Model file for the job. Use its own axes, mm. Face numbers are marked on the shaded views. A direction names the side the tool comes from. Coordinates: 2 decimals unless noted, no trailing zeros. Write each loop counter-clockwise with the first axis right and the second up, starting at its lowest first coordinate (ties: lowest second). Pieces come first, ordered by that corner, then holes. Notation, with made-up numbers: M -12.75,43.5 L 43.25,43.5 A19 cw 43.25,49.5 Z; hole C 25.25,39 d1. An arc over 180 degrees is marked long. Answer in a Markdown table with one row per item. Add a question column.
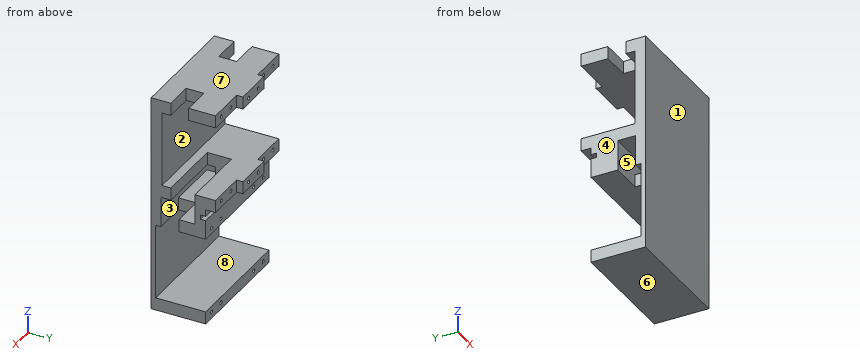
```python
from build123d import *

# Parameters (mm, degrees)
SKETCH1_W            = 66
SKETCH1_H            = 56
BOSS_EXTRUDE1_DEPTH  = 6
SKETCH2_W            = 66
SKETCH2_H            = 7
BOSS_EXTRUDE2_DEPTH  = 30
SKETCH4_W            = 22
SKETCH4_H            = 7
BOSS_EXTRUDE3_DEPTH  = 3.5
SKETCH6_R            = 1
CUT_EXTRUDE1_DEPTH   = 10
SKETCH15_W           = 66
SKETCH15_H           = 66
BOSS_EXTRUDE4_DEPTH  = 2.5
SKETCH16_W           = 66
SKETCH16_H           = 7
BOSS_EXTRUDE6_DEPTH  = 28
SKETCH17_R           = 1
CUT_EXTRUDE2_DEPTH   = 10
CUT_EXTRUDE3_REACH   = 9
SKETCH14_W           = 16
SKETCH14_H           = 10
CUT_EXTRUDE4_REACH   = 75
SKETCH19_W           = 18
SKETCH19_H           = 10
SKETCH24_W           = 66
SKETCH24_H           = 15
BOSS_EXTRUDE9_DEPTH  = 10
SKETCH27_W           = 38
SKETCH27_H           = 13.5
CUT_EXTRUDE9_DEPTH   = 17
SKETCH26_W           = 66
SKETCH26_H           = 3
BOSS_EXTRUDE10_DEPTH = 10
SKETCH28_W           = 66
SKETCH28_H           = 2.5
CUT_EXTRUDE10_DEPTH  = 3


with BuildPart() as part:
    # Sketch1 → Boss-Extrude1 (new body)
    with BuildSketch(Plane(origin=(0, 0, 0), x_dir=(1, 0, 0), z_dir=(0, 1, 0))):
        with Locations((33, 28)):
            Rectangle(SKETCH1_W, SKETCH1_H)
    boss_extrude1 = extrude(amount=BOSS_EXTRUDE1_DEPTH)

    # Sketch2 → Boss-Extrude2 (add)
    with BuildSketch(Plane(origin=(0, 6, 0), x_dir=(1, 0, 0), z_dir=(0, 1, 0))):
        with Locations((33, 52.5)):
            Rectangle(SKETCH2_W, SKETCH2_H)
    boss_extrude2 = extrude(amount=BOSS_EXTRUDE2_DEPTH)

    # Sketch4 → Boss-Extrude3 (add)
    with BuildSketch(Plane(origin=(0, 36, 0), x_dir=(1, 0, 0), z_dir=(0, 1, 0))):
        with Locations((33, 52.5)):
            Rectangle(SKETCH4_W, SKETCH4_H)
    boss_extrude3 = extrude(amount=BOSS_EXTRUDE3_DEPTH)

    # Sketch6 → Cut-Extrude1 (cut, symmetric)
    with BuildSketch(Plane(origin=(0, 36, 0), x_dir=(1, 0, 0), z_dir=(0, 1, 0))):
        with Locations((6, 52.25)):
            Circle(SKETCH6_R)
        with Locations((16, 52.25)):
            Circle(SKETCH6_R)
        with Locations((38, 52.25)):
            Circle(SKETCH6_R)
        with Locations((28, 52.25)):
            Circle(SKETCH6_R)
        with Locations((60, 52.25)):
            Circle(SKETCH6_R)
        with Locations((50, 52.25)):
            Circle(SKETCH6_R)
    cut_extrude1 = extrude(amount=CUT_EXTRUDE1_DEPTH, both=True, mode=Mode.SUBTRACT)

    # Mirror1: Boss-Extrude1, Boss-Extrude2, Boss-Extrude3, Cut-Extrude1 across plane
    add(boss_extrude1.mirror(Plane.XY.offset(-28)))
    add(boss_extrude2.mirror(Plane.XY.offset(-28)))
    add(boss_extrude3.mirror(Plane.XY.offset(-28)))
    add(cut_extrude1.mirror(Plane.XY.offset(-28)), mode=Mode.SUBTRACT)

    # Sketch15 → Boss-Extrude4 (add)
    with BuildSketch(Plane(origin=(0, 0, 0), x_dir=(1, 0, 0), z_dir=(0, 1, 0))):
        with Locations((33, 89)):
            Rectangle(SKETCH15_W, SKETCH15_H)
    extrude(amount=BOSS_EXTRUDE4_DEPTH)

    # Sketch16 → Boss-Extrude6 (add)
    with BuildSketch(Plane(origin=(0, 2.5, 0), x_dir=(1, 0, 0), z_dir=(0, 1, 0))):
        with Locations((33, 69.5)):
            Rectangle(SKETCH16_W, SKETCH16_H)
    boss_extrude6 = extrude(amount=BOSS_EXTRUDE6_DEPTH)

    # Sketch17 → Cut-Extrude2 (cut)
    with BuildSketch(Plane(origin=(0, 30.5, 0), x_dir=(1, 0, 0), z_dir=(0, 1, 0))):
        with Locations((6, 69.75)):
            Circle(SKETCH17_R)
        with Locations((16, 69.75)):
            Circle(SKETCH17_R)
        with Locations((50, 69.75)):
            Circle(SKETCH17_R)
        with Locations((60, 69.75)):
            Circle(SKETCH17_R)
    cut_extrude2 = extrude(amount=-CUT_EXTRUDE2_DEPTH, mode=Mode.SUBTRACT)

    # Mirror2: Boss-Extrude6, Cut-Extrude2 across plane
    add(boss_extrude6.mirror(Plane(origin=(0, 0, -94), x_dir=(1, 0, 0), z_dir=(0, 0, -1))))
    add(cut_extrude2.mirror(Plane(origin=(0, 0, -94), x_dir=(1, 0, 0), z_dir=(0, 0, -1))), mode=Mode.SUBTRACT)

    # Sketch14 → Cut-Extrude3 (cut, up to next)
    with BuildSketch(Plane(origin=(0, 0, -7), x_dir=(-1, 0, 0), z_dir=(0, 0, -1)), mode=Mode.PRIVATE) as cut_extrude3_sk1:
        with Locations((-8, 16)):
            Rectangle(SKETCH14_W, SKETCH14_H)
    cut_extrude3_tool1 = extrude(cut_extrude3_sk1.sketch, amount=-CUT_EXTRUDE3_REACH, mode=Mode.PRIVATE) & part.part
    add(cut_extrude3_tool1.solids().sort_by_distance((8, 16, -7))[0], mode=Mode.SUBTRACT)
    # Sketch14 → Cut-Extrude3 (cut, up to next)
    with BuildSketch(Plane(origin=(0, 0, -7), x_dir=(-1, 0, 0), z_dir=(0, 0, -1)), mode=Mode.PRIVATE) as cut_extrude3_sk2:
        with Locations((-58, 16)):
            Rectangle(SKETCH14_W, SKETCH14_H)
    cut_extrude3_tool2 = extrude(cut_extrude3_sk2.sketch, amount=-CUT_EXTRUDE3_REACH, mode=Mode.PRIVATE) & part.part
    add(cut_extrude3_tool2.solids().sort_by_distance((58, 16, -7))[0], mode=Mode.SUBTRACT)

    # Sketch19 → Cut-Extrude4 (cut, up to next)
    with BuildSketch(Plane(origin=(0, 0, -73), x_dir=(-1, 0, 0), z_dir=(0, 0, -1)), mode=Mode.PRIVATE) as cut_extrude4_sk1:
        with Locations((-9, 10.5)):
            Rectangle(SKETCH19_W, SKETCH19_H)
    cut_extrude4_tool1 = extrude(cut_extrude4_sk1.sketch, amount=-CUT_EXTRUDE4_REACH, mode=Mode.PRIVATE) & part.part
    add(cut_extrude4_tool1.solids().sort_by_distance((9, 10.5, -73))[0], mode=Mode.SUBTRACT)
    # Sketch19 → Cut-Extrude4 (cut, up to next)
    with BuildSketch(Plane(origin=(0, 0, -73), x_dir=(-1, 0, 0), z_dir=(0, 0, -1)), mode=Mode.PRIVATE) as cut_extrude4_sk2:
        with Locations((-57, 10.5)):
            Rectangle(SKETCH19_W, SKETCH19_H)
    cut_extrude4_tool2 = extrude(cut_extrude4_sk2.sketch, amount=-CUT_EXTRUDE4_REACH, mode=Mode.PRIVATE) & part.part
    add(cut_extrude4_tool2.solids().sort_by_distance((57, 10.5, -73))[0], mode=Mode.SUBTRACT)

    # Sketch24 → Boss-Extrude9 (add)
    with BuildSketch(Plane.XY.offset(-66)):
        with Locations((33, 23)):
            Rectangle(SKETCH24_W, SKETCH24_H)
    extrude(amount=BOSS_EXTRUDE9_DEPTH)

    # Sketch27 → Cut-Extrude9 (cut)
    with BuildSketch(Plane.XY.offset(-49)):
        with Locations((47, 17.75)):
            Rectangle(SKETCH27_W, SKETCH27_H)
    extrude(amount=-CUT_EXTRUDE9_DEPTH, mode=Mode.SUBTRACT)

    # Sketch26 → Boss-Extrude10 (add)
    with BuildSketch(Plane.XY.offset(-66)):
        with Locations((33, 4)):
            Rectangle(SKETCH26_W, SKETCH26_H)
    extrude(amount=BOSS_EXTRUDE10_DEPTH)

    # Sketch28 → Cut-Extrude10 (cut)
    with BuildSketch(Plane(origin=(0, 30.5, 0), x_dir=(1, 0, 0), z_dir=(0, 1, 0))):
        with Locations((33, 61)):
            Rectangle(SKETCH28_W, SKETCH28_H)
    extrude(amount=-CUT_EXTRUDE10_DEPTH, mode=Mode.SUBTRACT)


solid = part.part
```
1) Slice it at A-A (y = 8.5). Give the cut face in (x, z), then the cut area to 3 significant figures.
2) Which spindle directions (+Z, -Z, +X, -X, +Y, -Y) get a long thin tool onto all of the face, cutting with end or side? Do the marked faces 1, 2, 3, 4 and 5. Say none if no direction does.
3) Slice it at C-C (z = -42). Give the cut face in (x, y), then the cut area to 3 significant figures.
4) Two-plate mould, pull along Z, no slides. Class the marked faces 6, 7 and 8: released by +Z, released by -Z, zero draft, split by the parting line, or undercut.
5) Drill centre lines: probe 1 along Z at (x, y) = (38, 30); probe 2 along Z at (x, y) = (28, 33); probe 3 along Z at (x, y) = (3, 29). Where is each one in solid material? Low to high.
6) Flat gauge pins, fed straight in: pin 1 Ø3 at (x, z) = (60, -3.75) entering from +Y; pin 2 Ø6 at (y, z) = (10, -60.5) entering from -X; pin 3 Ø0.6 at (x, z) = (59.5, -118) entering from +Y; pin 4 Ø2 at (y, z) = (18, -2) entering from +X. Where does each tip first touch, or does it go through?
7) Slice it at B-B (x = 57). Count the separate pieces of the cut face and the enclosed holes in it, then the cut area to 3 significant figures.
8) Slice it at D-D (z = -75). Give the cut face in (x, y).
Ans:
| question | item | result |
|---|---|---|
| 1 | outline | M 0,-122 L 66,-122 L 66,-115 L 0,-115 Z; M 0,-56 L 66,-56 L 66,-49 L 0,-49 Z; M 0,-7 L 66,-7 L 66,0 L 0,0 Z; M 18,-73 L 48,-73 L 48,-66 L 18,-66 Z |
| 1 | area | 1,600 mm2 |
| 2 | face 1 | +Z, -Z, +X, -X, -Y |
| 2 | face 2 | +X, -X, +Y |
| 2 | face 3 | none |
| 2 | face 4 | +Z, -Z, -X, +Y, -Y |
| 2 | face 5 | -X |
| 3 | outline | M 0,0 L 66,0 L 66,6 L 0,6 Z |
| 3 | area | 396 mm2 |
| 4 | face 6 | released by -Z |
| 4 | face 7 | released by +Z |
| 4 | face 8 | undercut |
| 5 | probe 1 | z = -122 to -115, -73 to -62.25, -59.75 to -53.25, -51.25 to -49, -7 to -4.75, -2.75 to 0 |
| 5 | probe 2 | z = -56 to -53.25, -51.25 to -49, -7 to -4.75, -2.75 to 0 |
| 5 | probe 3 | z = -122 to -115, -73 to -62.25, -59.75 to -49, -7 to 0 |
| 6 | pin 1 | stops at y = 36 |
| 6 | pin 2 | passes through |
| 6 | pin 3 | stops at y = 20.5 |
| 6 | pin 4 | stops at x = 50 |
| 7 | separate pieces | 3 |
| 7 | enclosed holes | 0 |
| 7 | area | 1,160 mm2 |
| 8 | outline | M 0,0 L 66,0 L 66,2.5 L 0,2.5 Z |
